```python
from build123d import *

# Parameters (mm, degrees)
ESQUISSE1_R             = 22.5
BOSS_EXTRU_1_DEPTH      = 3
ESQUISSE2_R             = 14.5
BOSS_EXTRU_2_DEPTH      = 6.5
ESQUISSE3_R             = 2
ESQUISSE3_R_2           = 3.1
ENL_V_MAT_EXTRU_1_DEPTH = 34.207679835


with BuildPart() as part:
    # Esquisse1 → Boss.-Extru.1 (new body)
    with BuildSketch(Plane.XY):
        Circle(ESQUISSE1_R)
    extrude(amount=BOSS_EXTRU_1_DEPTH)

    # Esquisse2 → Boss.-Extru.2 (add)
    with BuildSketch(Plane.XY.offset(3)):
        with Locations(Location((0, 0, 0), (0, 0, 180))):
            Circle(ESQUISSE2_R)
    extrude(amount=BOSS_EXTRU_2_DEPTH)

    # Esquisse3 → Enlèv. mat.-Extru.1 (cut, through all)
    with BuildSketch(Plane.XY.offset(9.5)):
        with Locations((8.660254038, 5)):
            Circle(ESQUISSE3_R)
        with Locations((-8.660254038, 5)):
            Circle(ESQUISSE3_R)
        with Locations((0, -10)):
            Circle(ESQUISSE3_R)
        Circle(ESQUISSE3_R_2)
    extrude(amount=-ENL_V_MAT_EXTRU_1_DEPTH, mode=Mode.SUBTRACT)


solid = part.part
```
Can you work these out from the model? Positions are in its coordinate system, mm. A direction names the side the tool comes from. Coordinates: 2 decimals unless noted, no trailing zeros. Order: outer loops, then holes, each group sorted by start corner. A loop starts at its lowest first (then second) coordinate and runs counter-clockwise, first axis right, second up. Notation, with made-up numbers: (-26, -20) -> (6, -20) arc R24 cw to (6, -9) -> close; hole circle Ø8 at (-16, 68). An arc over 180 degrees is marked (long way). Write each question's results on one line, items separated by ' | '.
Item 1: If I drill on line 1 along Y through (x, z) = (0, 0.5); line 2 along Z through (x, y) = (4.5, -20); line 3 along Y through (x, z) = (8, 3.25), over which ranges is the centre line in solid material (lowest first)?
Results are:
line 1: -22.5 to -12, -8 to -3.1, 3.1 to 22.5 | line 2: 0 to 3 | line 3: -12.09 to 3.11, 6.89 to 12.09
Item 2: I want a section at A-A, the plane x = 0. Write out the boundary of the cut face in (y, z).
Results are:
outline: (-22.5, 0) -> (-12, 0) -> (-12, 9.5) -> (-14.5, 9.5) -> (-14.5, 3) -> (-22.5, 3) -> close; (-8, 0) -> (-3.1, 0) -> (-3.1, 9.5) -> (-8, 9.5) -> close; (3.1, 0) -> (22.5, 0) -> (22.5, 3) -> (14.5, 3) -> (14.5, 9.5) -> (3.1, 9.5) -> close
Item 3: Which directions (+Z, -Z, +X, -X, +Y, -Y) give clear straight access to the entire face, cutting with the end or side of a thin tool? Please do faces 4 (the face through (0, -15, 3)), 5 (the face through (0, -5, 0)).
Results are:
face 4: +Z | face 5: -Z, +X, -X, +Y, -Y
Item 4: If we mould it in two halves opening along X, with no side actions, what happens to faces 1 (the face through (0.2, -3.4, 9.5)), 2 (the face through (1.43, -2.75, 4.82)), 3 (the face through (-6.691, 12.864, 6.204))? For each: +X half, -X half, draft (parallel to the pull), parting line (faces both ways), or undercut.
Results are:
face 1: draft | face 2: undercut | face 3: parting line
Item 5: I want a section at B-B, the plane y = 0. Write out the boundary of the cut face in (x, z).
Results are:
outline: (-22.5, 0) -> (-3.1, 0) -> (-3.1, 9.5) -> (-14.5, 9.5) -> (-14.5, 3) -> (-22.5, 3) -> close; (3.1, 0) -> (22.5, 0) -> (22.5, 3) -> (14.5, 3) -> (14.5, 9.5) -> (3.1, 9.5) -> close
Item 6: I'm going to push flat-ended pins straight in: pin 1 Ø2 at (y, z) = (14, 3) entering from -X; pin 2 Ø4 at (y, z) = (17.5, 4.5) entering from +X; pin 3 Ø3 at (y, z) = (12, 7) entering from +X. Where does each tip first touch, or does it pass through?
Results are:
pin 1: x = -18.36 | pin 2: x = 15.64 | pin 3: x = 10
Item 7: I want a section at C-C, the plane x = -9.5. Write out the boundary of the cut face in (y, z), then the cut area to 3 significant figures.
Results are:
outline: (-20.4, 0) -> (3.18, 0) -> (3.18, 9.5) -> (-10.95, 9.5) -> (-10.95, 3) -> (-20.4, 3) -> close; (6.82, 0) -> (20.4, 0) -> (20.4, 3) -> (10.95, 3) -> (10.95, 9.5) -> (6.82, 9.5) -> close | area: 230 mm²
Item 8: I want a section at D-D, the plane z = 1. Write out the boundary of the cut face in (x, y), then the cut area to 3 significant figures.
Results are:
outline: circle Ø45 at (0, 0); hole circle Ø4 at (-8.66, 5); hole circle Ø6.2 at (0, 0); hole circle Ø4 at (0, -10); hole circle Ø4 at (8.66, 5) | area: 1,520 mm²
